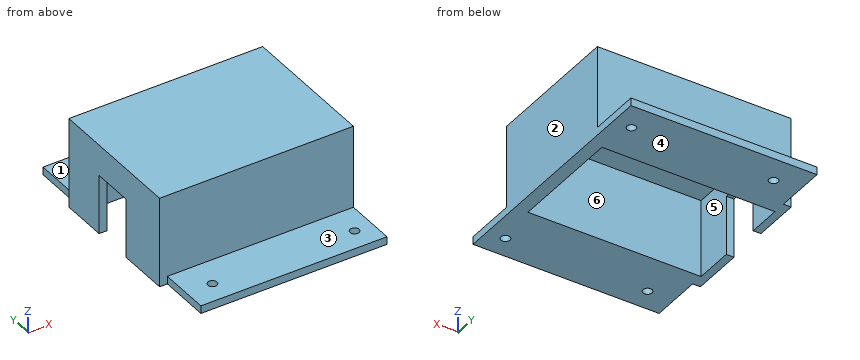
Autodesk Fusion 360 part; units mm, degrees
sketch "Sketch1" plane through (0, 0, 0) normal (0, 0, 1) x (1, 0, 0)
  line L0 (70, 0) -> (70, 54)
  line L1 (70, 54) -> (0, 54)
  line L2 (0, 54) -> (0, 0)
  line L3 (5, 49) -> (65, 49)
  line L4 (65, 49) -> (65, 5)
  line L5 (65, 5) -> (5, 5)
  line L6 (5, 5) -> (5, 49)
  line L7 (0, 0) -> (70, 0)
  line L8 (0, 54) -> (70, 54)
  line L9 (70, 54) -> (70, 74)
  line L10 (70, 74) -> (0, 74)
  line L11 (0, 74) -> (0, 54)
  line L12 (0, 0) -> (70, 0)
  line L13 (70, 0) -> (70, -20)
  line L14 (70, -20) -> (0, -20)
  line L15 (0, -20) -> (0, 0)
  dimension "d1" = 54
  dimension "d2" = 70
  dimension "d3" = 5
  dimension "d4" = 5
  dimension "d5" = 5
  dimension "d11" = 5
  dimension "d12" = 20
  dimension "d13" = 20
extrude "Extrude1" add sketch "Sketch1" along normal blind 30 contours L0 L1 L2 L7 L8 L12
extrude "Extrude2" add sketch "Sketch1" along normal blind 3 contours L7 L12 L13 L14 L15 | L1 L8 L9 L10 L11
sketch "Sketch3" plane through (0, 0, 30) normal (0, 0, 1) x (-1, 0, 0)
  line L0 (-65, -5) -> (-5, -5)
  line L1 (-5, -5) -> (-5, -49)
  line L2 (-5, -49) -> (-65, -49)
  line L3 (-65, -49) -> (-65, -5)
  line L4 (0, -54) -> (0, 0)
  line L5 (0, 0) -> (-70, 0)
  line L6 (-70, 0) -> (-70, -54)
  line L7 (-70, -54) -> (0, -54)
  line L8 (0, -54) -> (-70, -54)
  line L9 (-70, -54) -> (-70, 0)
  line L10 (-70, 0) -> (0, 0)
  line L11 (0, 0) -> (0, -54)
extrude "Extrude3" add sketch "Sketch3" along normal blind 5 contours L0 L1 L2 L3 | L4 L5 L6 L7 L8 L9 L10 L11
sketch "Sketch4" plane through (0, 0, 3) normal (0, 0, 1) x (-1, 0, 0)
  line L0 (0, -74) -> (0, -54)
  line L1 (0, -54) -> (-70, -54)
  line L2 (-70, -54) -> (-70, -74)
  line L3 (-70, -74) -> (0, -74)
  circle A0 centre (-8, -63.531) radius 1.75
  circle A1 centre (-63, -63.531) radius 1.75
  circle A2 centre (-8, 11.469) radius 1.75
  circle A3 centre (-63, 11.469) radius 1.75
  line L4 (0, -74) -> (0, -54)
  line L5 (-70, -74) -> (0, -74)
  dimension "d18" = 3.5
  dimension "d21" = -55
  dimension "d22" = 75
  dimension "d23" = 8
  dimension "d24" = 10.469
extrude "Extrude4" cut sketch "Sketch4" against normal blind 3 contours A0 | A1 | A2 | A3
sketch "Sketch5" plane through (0, 0, 0) normal (-1, 0, 0) x (0, -1, 0)
  line L0 (-74, 0) -> (20, 0)
  line L1 (20, 0) -> (20, 3)
  line L2 (20, 3) -> (0, 3)
  line L3 (0, 3) -> (0, 35)
  line L4 (0, 35) -> (-54, 35)
  line L5 (-54, 35) -> (-54, 3)
  line L6 (-54, 3) -> (-74, 3)
  line L7 (-74, 3) -> (-74, 0)
  line L8 (-5, 0) -> (-49, 0)
  line L9 (-49, 0) -> (-49, 30)
  line L10 (-49, 30) -> (-5, 30)
  line L11 (-5, 30) -> (-5, 0)
  dimension "d27" = 5
  dimension "d28" = 5
  dimension "d33" = 5
extrude "Extrude5" cut sketch "Sketch5" against normal blind 5 contours L0 L8 L9 L10 L11
extrude "Extrude6" add 1 faces at (0, 34.3333, 33.3333) along direction (-1, 0, 0) blind 2
sketch "Sketch7" plane through (-2, 0, 0) normal (-1, 0, 0) x (0, -1, 0)
  line L0 (-5, 30) -> (-5, 0)
  line L1 (-5, 0) -> (20, 0)
  line L2 (20, 0) -> (20, 3)
  line L3 (20, 3) -> (0, 3)
  line L4 (0, 3) -> (0, 35)
  line L5 (0, 35) -> (-54, 35)
  line L6 (-54, 35) -> (-54, 3)
  line L7 (-54, 3) -> (-74, 3)
  line L8 (-74, 3) -> (-74, 0)
  line L9 (-74, 0) -> (-49, 0)
  line L10 (-49, 0) -> (-49, 30)
  line L11 (-49, 30) -> (-5, 30)
  line L12 (-54, 35) -> (0, 35)
  line L13 (0, 35) -> (0, 0)
  line L14 (0, 0) -> (-54, 0)
  line L15 (-54, 0) -> (-54, 35)
extrude "Extrude7" add sketch "Sketch7" along normal blind 3 contours L0 L1 L4 L5 L6 L9 L10 L11 L12 L13 L14 L15 | L0 L10 L11 L14
sketch "Sketch8" plane through (-5, 0, 0) normal (-1, 0, 0) x (0, -1, 0)
  line L0 (-54, 0) -> (0, 0)
  line L1 (0, 0) -> (0, 35)
  line L2 (0, 35) -> (-54, 35)
  line L3 (-54, 35) -> (-54, 0)
  line L4 (-36, 0) -> (-20, 0)
  line L5 (-20, 0) -> (-20, 23)
  line L6 (-20, 23) -> (-36, 23)
  line L7 (-36, 23) -> (-36, 0)
  line L8 (-74, 3) -> (-74, 0)
  line L9 (20, 0) -> (20, 3)
  dimension "d39" = 38
  dimension "d40" = 40
  dimension "d41" = 23
extrude "Extrude8" cut sketch "Sketch8" against normal blind 3 contours L0 L4 L5 L6 L7
Source: CAD feature listing. Evaluate the final solid. Frame: model axes, mm. Face numbers are marked on the shaded views. A direction names the side the tool comes from. Coordinates: 2 decimals unless noted, no trailing zeros. Loops run counter-clockwise (first coordinate to the right, second up) from the corner with the lowest first, then second, coordinate; pieces in that order, holes last. Notation, with made-up numbers: (64.25, -33.75) -> (118.25, -33.75) arc R30 cw to (118.25, -7.75) -> close; hole circle Ø3 at (-35.75, 37.5). An arc over 180 degrees is marked (long way). One line per item, written item: value. Start each with the question number.
Q1. Set-up query: the marked faces 1, 2 and 3. Return all of +Z, -Z, +X, -X, +Y, -Y with unobstructed straight access to the full face (end or side cutting, diameter ignored); none if empty.
Q2. Line query: line 1 along Y through (x, z) = (63, 2); line 2 along X through (y, z) = (24.5, 28); line 3 along Y through (x, z) = (55, 5.5). Output: solid intervals per line, ascending.
Q3. Mould query, pull axis Y, two halves, no side actions, for the marked faces 4, 5 and 6. Classes: pulls with the +Y half, pulls with the -Y half, needs draft (parallel to the pull), parting line crosses it, or undercut.
Q4. Section query B-B, the plane z = 13. Return the cut outline in (x, y).
Q5. Section query A-A, the plane x = 8. Return the cut outline in (y, z), and give its area (3 significant figures).
Q6. Section query C-C, the plane y = 24. Return the cut outline in (x, z), and give its area (3 significant figures).
Q7. Contact query for flat-ended pins moving along their axis: P1, Ø4, axis at x = 9, z = 25, coming from the -Y side; P2, Ø3, axis at x = 8, y = -11.469, coming from the +Z side; P3, Ø1, axis at x = 8.5, z = 31, coming from the +Y side; P4, Ø3.5, axis at y = -6.5, z = 1.5, coming from the -X side. Output: stop coordinate, or through.
Q8. Section query D-D, the plane x = 31.5. Return the cut outline in (y, z).
Results:
1. face 1: +Z, +X, -X, +Y
1. face 2: +Z, -Z, +X, +Y, -Y
1. face 3: +Z, +X, -X, -Y
2. line 1: -20 to -13.22, -9.72 to 5, 49 to 61.78, 65.28 to 74
2. line 2: -5 to -2, 65 to 70
2. line 3: 0 to 5, 49 to 54
3. face 4: needs draft
3. face 5: undercut
3. face 6: undercut
4. outline: (-5, 0) -> (70, 0) -> (70, 54) -> (-5, 54) -> (-5, 36) -> (-2, 36) -> (-2, 49) -> (65, 49) -> (65, 5) -> (-2, 5) -> (-2, 20) -> (-5, 20) -> close
5. outline: (-20, 0) -> (-13.22, 0) -> (-13.22, 3) -> (-20, 3) -> close; (-9.72, 0) -> (5, 0) -> (5, 30) -> (49, 30) -> (49, 0) -> (61.78, 0) -> (61.78, 3) -> (54, 3) -> (54, 35) -> (0, 35) -> (0, 3) -> (-9.72, 3) -> close; (65.28, 0) -> (74, 0) -> (74, 3) -> (65.28, 3) -> close
5. area: 669 mm^2
6. outline: (-5, 23) -> (-2, 23) -> (-2, 30) -> (65, 30) -> (65, 0) -> (70, 0) -> (70, 35) -> (-5, 35) -> close
6. area: 546 mm^2
7. P1: y = 0
7. P2: through
7. P3: y = 54
7. P4: x = -2
8. outline: (-20, 0) -> (5, 0) -> (5, 30) -> (49, 30) -> (49, 0) -> (74, 0) -> (74, 3) -> (54, 3) -> (54, 35) -> (0, 35) -> (0, 3) -> (-20, 3) -> close
